from build123d import *

# Parameters (mm, degrees)
MODEL_R             = 4
MODEL_W             = 6
MODEL_H             = 10.5
BOSS_EXTRUDE1_DEPTH = 3


with BuildPart() as part:
    # Model → Boss-Extrude1 (new body)
    with BuildSketch(Plane.XY):
        Polygon((-215.742718731, 39.275539879), (-157.242718731, 39.275539879), (-157.242718731, 42.275539879), (-137.242718731, 42.275539879), (-137.242718731, 39.275539879), (-125.742718731, 39.275539879), (-125.742718731, 100.275539879), (-95.742718731, 100.275539879), (-95.742718731, 39.275539879), (-73.742718731, 39.275539879), (-73.742718731, 42.275539879), (-63.742718731, 42.275539879), (-63.742718731, 39.275539879), (-55.742718731, 39.275539879), (-55.742718731, 69.275539879), (-58.742718731, 69.275539879), (-58.742718731, 99.275539879), (-55.742718731, 99.275539879), (-55.742718731, 129.275539879), (-132.242718731, 129.275539879), (-132.242718731, 128.275539879), (-162.242718731, 128.275539879), (-162.242718731, 129.275539879), (-235.742718731, 129.275539879), (-235.742718731, 99.275539879), (-238.742718731, 99.275539879), (-238.742718731, 69.275539879), (-235.742718731, 69.275539879), (-235.742718731, 39.275539879), (-227.742718731, 39.275539879), (-227.742718731, 42.275539879), (-217.742718731, 42.275539879), (-217.742718731, 39.275539879), align=None)
        with Locations((-142.742718731, 112.275539879)):
            Circle(MODEL_R, mode=Mode.SUBTRACT)
        with Locations((-133.742718731, 74.525539879)):
            Rectangle(MODEL_W, MODEL_H, mode=Mode.SUBTRACT)
    extrude(amount=BOSS_EXTRUDE1_DEPTH)


solid = part.part
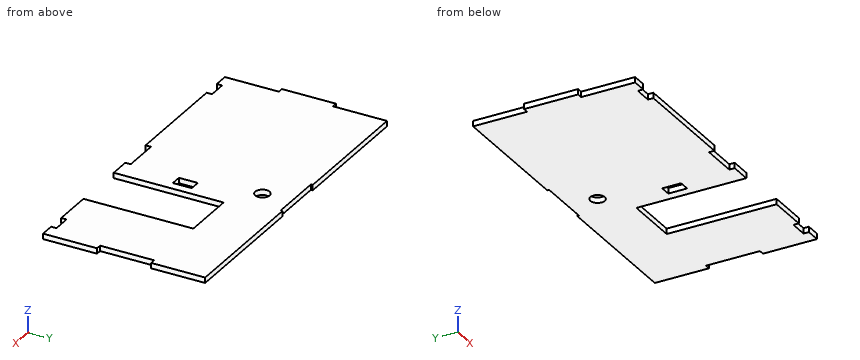
Part model, mm, in its own coordinate system. Coordinates: 2 decimals unless noted, no trailing zeros. Write each loop counter-clockwise with the first axis right and the second up, starting at its lowest first coordinate (ties: lowest second). Pieces come first, ordered by that corner, then holes. Notation, with made-up numbers: M -30.75,47.5 L 4.25,47.5 A32 cw 4.25,79.5 Z; hole C -8,85.5 d1. An arc over 180 degrees is marked long. Return JSON: item names as keys, results as strings.
1. Probe L1, parallel to X at y = 70, z = 2.2; L2, parallel to X at y = 87.5, z = 2.5; L3, parallel to X at y = 49.5, z = 0.8. List the from-to ranges inside material, lowest first.
Determined:
{"L1": "-238.74 to -136.74, -130.74 to -125.74, -95.74 to -58.74", "L2": "-238.74 to -125.74, -95.74 to -58.74", "L3": "-235.74 to -125.74, -95.74 to -55.74"}
2. Saw through at A-A, the plane y = 82.5. Write the cut outline in (x, z).
Determined:
{"outline": "M -238.74,0 L -125.74,0 L -125.74,3 L -238.74,3 Z; M -95.74,0 L -58.74,0 L -58.74,3 L -95.74,3 Z"}
3. Saw through at D-D, the plane y = 122.5. Write the cut outline in (x, z).
Determined:
{"outline": "M -235.74,0 L -55.74,0 L -55.74,3 L -235.74,3 Z"}
4. Saw through at B-B, the plane x = -151.5. Write the cut outline in (y, z).
Determined:
{"outline": "M 42.28,0 L 128.28,0 L 128.28,3 L 42.28,3 Z"}
5. Flat gauge pins, fed straight in: pin 1 Ø0.9 at (x, z) = (-225, 1) entering from -Y; pin 2 Ø0.9 at (y, z) = (74, 1) entering from +X; pin 3 Ø0.9 at (x, z) = (-133.5, 1.5) entering from +Y; pin 4 Ø7 at (x, y) = (-142.74, 112.28) entering from -Z. Where does each tip first touch, or does it go through?
Determined:
{"pin 1": "y = 42.28", "pin 2": "x = -58.74", "pin 3": "y = 128.28", "pin 4": "through"}
6. Saw through at C-C, the plane z = 1.8. Count the separate pieces of the cut face and the enclosed holes in it, then the cut area to 3 significant figures.
Determined:
{"separate pieces": "1", "enclosed holes": "2", "area": "14,100 mm²"}
